from build123d import *
from build123d.topology import SkipClean

# Parameters (mm, degrees)
BOSS_EXTRUDE1_DEPTH = 2
SKETCH2_R           = 1.000000794
CUT_EXTRUDE1_DEPTH  = 2
SKETCH3_R           = 4.5
BOSS_EXTRUDE2_DEPTH = 5.08
SKETCH4_R           = 2.75
CUT_EXTRUDE2_DEPTH  = 3.5
SKETCH5_R           = 3.25
CUT_EXTRUDE3_DEPTH  = 3.25
SKETCH7_R           = 6.724332425
BOSS_EXTRUDE3_DEPTH = 0.5
SKETCH8_W           = 14.5
SKETCH8_H           = 1.25
SKETCH8_H_2         = 1.25000004
BOSS_EXTRUDE4_DEPTH = 0.5
SKETCH6_R           = 2
CUT_EXTRUDE4_DEPTH  = 30.338041851
SKETCH15_R          = 3.25
CUT_EXTRUDE5_DEPTH  = 3.75


# Read off the part's stored shape, not the designer's step: Mirror3
with BuildPart() as part:
    # Sketch1 → Boss-Extrude1 (new body)
    with BuildSketch(Plane(origin=(0, 0, 0), x_dir=(1, 0, 0), z_dir=(0, 1, 0))):
        with BuildLine():
            Line((-24.656541995, 4.026414392), (-0.733072501, 6.659779954))
            ThreePointArc((-0.733072501, 6.659779954), (0, 6.695526614), (0.733072501, 6.659779954))
            Line((0.733072501, 6.659779954), (24.656541995, 4.026414392))
            ThreePointArc((24.656541995, 4.026414392), (28.264069964, 0), (24.656541995, -4.026414392))
            Line((24.656541995, -4.026414392), (0.733072501, -6.659779954))
            ThreePointArc((0.733072501, -6.659779954), (0, -6.695526614), (-0.733072501, -6.659779954))
            Line((-0.733072501, -6.659779954), (-24.656541995, -4.026414392))
            ThreePointArc((-24.656541995, -4.026414392), (-28.264069964, 0), (-24.656541995, 4.026414392))
        make_face()
    extrude(amount=BOSS_EXTRUDE1_DEPTH)

    # Sketch2 → Cut-Extrude1 (cut)
    with BuildSketch(Plane(origin=(0, 2, 0), x_dir=(1, 0, 0), z_dir=(0, 1, 0))):
        with Locations(Location((-24.320001144, 0, 0), (0, 0, 270))):
            Circle(SKETCH2_R)
        with Locations(Location((-21.222128244, 0, 0), (0, 0, 270))):
            Circle(SKETCH2_R)
        with Locations(Location((-18.117543648, 0, 0), (0, 0, 270))):
            Circle(SKETCH2_R)
        with Locations(Location((-15.019999932, 0, 0), (0, 0, 270))):
            Circle(SKETCH2_R)
        with Locations(Location((-11.919999782, 0, 0), (0, 0, 270))):
            Circle(SKETCH2_R)
        with Locations(Location((24.320001144, 0, 0), (0, 0, 90))):
            Circle(SKETCH2_R)
        with Locations(Location((21.222128244, 0, 0), (0, 0, 90))):
            Circle(SKETCH2_R)
        with Locations(Location((18.117543648, 0, 0), (0, 0, 90))):
            Circle(SKETCH2_R)
        with Locations(Location((15.019999932, 0, 0), (0, 0, 90))):
            Circle(SKETCH2_R)
        with Locations(Location((11.919999782, 0, 0), (0, 0, 90))):
            Circle(SKETCH2_R)
    extrude(amount=-CUT_EXTRUDE1_DEPTH, mode=Mode.SUBTRACT)

    # Sketch3 → Boss-Extrude2 (add)
    with BuildSketch(Plane(origin=(0, 2, 0), x_dir=(1, 0, 0), z_dir=(0, 1, 0))):
        with Locations(Location((0, 0, 0), (0, 0, 270))):
            Circle(SKETCH3_R)
    extrude(amount=BOSS_EXTRUDE2_DEPTH)

    # Sketch4 → Cut-Extrude2 (cut)
    with BuildSketch(Plane(origin=(0, 7.08, 0), x_dir=(1, 0, 0), z_dir=(0, 1, 0))):
        with Locations(Location((0, 0, 0), (0, 0, 270))):
            Circle(SKETCH4_R)
    extrude(amount=-CUT_EXTRUDE2_DEPTH, mode=Mode.SUBTRACT)

    # Sketch5 → Cut-Extrude3 (cut)
    with BuildSketch(Plane.XZ):
        with Locations(Location((0, 0, 0), (0, 0, 270))):
            Circle(SKETCH5_R)
    extrude(amount=-CUT_EXTRUDE3_DEPTH, mode=Mode.SUBTRACT)

    # Sketch7 → Boss-Extrude3 (add)
    with BuildSketch(Plane.XZ):
        with Locations(Location((0, 0, 0), (0, 0, 78.843263662))):
            Circle(SKETCH7_R)
    extrude(amount=BOSS_EXTRUDE3_DEPTH)

    # Sketch8 → Boss-Extrude4 (add)
    with BuildSketch(Plane.XZ):
        Rectangle(SKETCH8_W, SKETCH8_H)
        with Locations((0, -4.843845819)):
            Rectangle(SKETCH8_W, SKETCH8_H_2)
        with Locations((0, 4.843845819)):
            Rectangle(SKETCH8_W, SKETCH8_H_2)
    extrude(amount=BOSS_EXTRUDE4_DEPTH)

    # Sketch13 → Cut-Loft1 section 0
    with BuildSketch(Plane.XY.offset(-4.218845799)):
        with BuildLine():
            Line((-7.25, 0), (-5.236218739, -0.5))
            Line((-5.236218739, -0.5), (-7.25, -0.5))
            Line((-7.25, -0.5), (-7.25, 0))
        make_face()
    # Sketch12 → Cut-Loft1 section 1
    with BuildSketch(Plane(origin=(0, 0, -5.468845839), x_dir=(-1, 0, 0), z_dir=(0, 0, -1))):
        with BuildLine():
            Line((3.912591436, -0.5), (7.25, -0.5))
            Line((7.25, -0.5), (7.25, 0))
            Line((7.25, 0), (3.912591436, -0.5))
        make_face()
    cut_loft1 = loft(mode=Mode.SUBTRACT)

    # Mirror1: Cut-Loft1 across plane
    add(cut_loft1.mirror(Plane.XY), mode=Mode.SUBTRACT)

    # Mirror2: Cut-Loft1 across plane
    add(cut_loft1.mirror(Plane(origin=(0, 0, 0), x_dir=(0, 0, 1), z_dir=(1, 0, 0))), mode=Mode.SUBTRACT)

    # Mirror3
    split(bisect_by=Plane.XY, keep=Keep.BOTTOM)

    # Mirror3 2: part across plane


with BuildPart() as part_1:
    with SkipClean():  # the faces are left unmerged after this step: merging them gives an invalid solid
        add(part.part)
        add(part.part.mirror(Plane.XY))

    # Sketch10 → Cut-Loft2 section 0
    with SkipClean():  # the faces are left unmerged after this step: merging them gives an invalid solid
        with BuildSketch(Plane(origin=(0, 0, -0.625), x_dir=(-1, 0, 0), z_dir=(0, 0, -1))):
            with BuildLine():
                Line((7.25, -0.5), (6.695223787, -0.5))
                Line((6.695223787, -0.5), (7.25, 0))
                Line((7.25, 0), (7.25, -0.5))
            make_face()
        # Sketch14 → Cut-Loft2 section 1
        with BuildSketch(Plane.XY.offset(0.625)):
            with BuildLine():
                Line((-7.25, 0), (-6.695223787, -0.5))
                Line((-6.695223787, -0.5), (-7.25, -0.5))
                Line((-7.25, -0.5), (-7.25, 0))
            make_face()
        cut_loft2 = loft(mode=Mode.SUBTRACT)

    # Mirror5: Cut-Loft2 across plane
    with SkipClean():  # the faces are left unmerged after this step: merging them gives an invalid solid
        add(cut_loft2.mirror(Plane(origin=(0, 0, 0), x_dir=(0, 0, 1), z_dir=(1, 0, 0))), mode=Mode.SUBTRACT)

    # Sketch6 → Cut-Extrude4 (cut, through all)
    with SkipClean():  # the faces are left unmerged after this step: merging them gives an invalid solid
        with BuildSketch(Plane(origin=(0, 3.58, 0), x_dir=(1, 0, 0), z_dir=(0, 1, 0))):
            with Locations(Location((0, 0, 0), (0, 0, 270))):
                Circle(SKETCH6_R)
        extrude(amount=-CUT_EXTRUDE4_DEPTH, mode=Mode.SUBTRACT)

    # Sketch15 → Cut-Extrude5 (cut)
    with SkipClean():  # the faces are left unmerged after this step: merging them gives an invalid solid
        with BuildSketch(Plane.XZ.offset(0.5)):
            with Locations(Location((0, 0, 0), (0, 0, 270))):
                Circle(SKETCH15_R)
        extrude(amount=-CUT_EXTRUDE5_DEPTH, mode=Mode.SUBTRACT)


solid = part_1.part
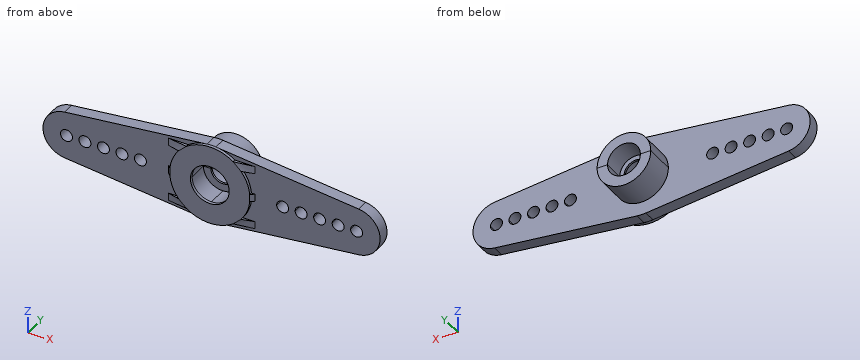
Work out the finished part from the listing and answer in its coordinate system (mm). Round coordinates to 2 decimals unless told otherwise and drop trailing zeros. Write each loop counter-clockwise with the first axis right and the second up, starting at its lowest first coordinate (ties: lowest second). Pieces come first, ordered by that corner, then holes. Notation, with made-up numbers: M -12.75,81.25 L -3.75,81.25 A24 cw -3.75,119.25 Z; hole C -7,-32 d1. An arc over 180 degrees is marked long. Use a Markdown table: item, result.
1) The part is cut by section B-B on x = 15. Give the vertices of the cut face in (y, z).
Taken from the geometry:
| item | result |
|---|---|
| outline | M 0,-5.09 L 2,-5.09 L 2,-1 L 0,-1 Z; M 0,1 L 2,1 L 2,5.09 L 0,5.09 Z |
2) The part is cut by section C-C on y = 4.5. Give the vertices of the cut face in (x, z), plus the area to 3 significant figures.
Taken from the geometry:
| item | result |
|---|---|
| outline | C 0,0 d9; hole C 0,0 d5.5 |
| area | 39.9 mm2 |
3) Flat-ended cylindrical pins translate along their axes: pin 1 (3 mm diameter, centred on x = -20, y = 4.5, fed in from +Z); pin 2 (3 mm diameter, centred on x = -21.22, z = 0, fed in from -Y); pin 3 (1.5 mm diameter, centred on y = 3.5, z = -4.5, fed in from -X); pin 4 (2 mm diameter, centred on x = -13, z = -5, fed in from +Y). Find the tip coordinate at first contact, or state that the pin passes through.
Taken from the geometry:
| item | result |
|---|---|
| pin 1 | passes through |
| pin 2 | stops at y = 0 |
| pin 3 | stops at x = -2.49 |
| pin 4 | stops at y = 2 |
4) Consider line 1 (Z direction, x = 0, y = 3.4); line 2 (X direction, y = 6.25, z = 0); line 3 (Y direction, x = 4.5, z = -4.5). Determine where each line is inside the solid, lowest interval first. Write a range as [from, to].
Taken from the geometry:
| item | result |
|---|---|
| line 1 | z = [-4.5, -2], [2, 4.5] |
| line 2 | x = [-4.5, -2.75], [2.75, 4.5] |
| line 3 | y = [-0.5, 2] |
5) The part is cut by section A-A on y = 1. State how many separate pieces and enclosed holes the cut face has, plus the area to 3 significant figures.
Taken from the geometry:
| item | result |
|---|---|
| separate pieces | 1 |
| enclosed holes | 11 |
| area | 511 mm2 |
